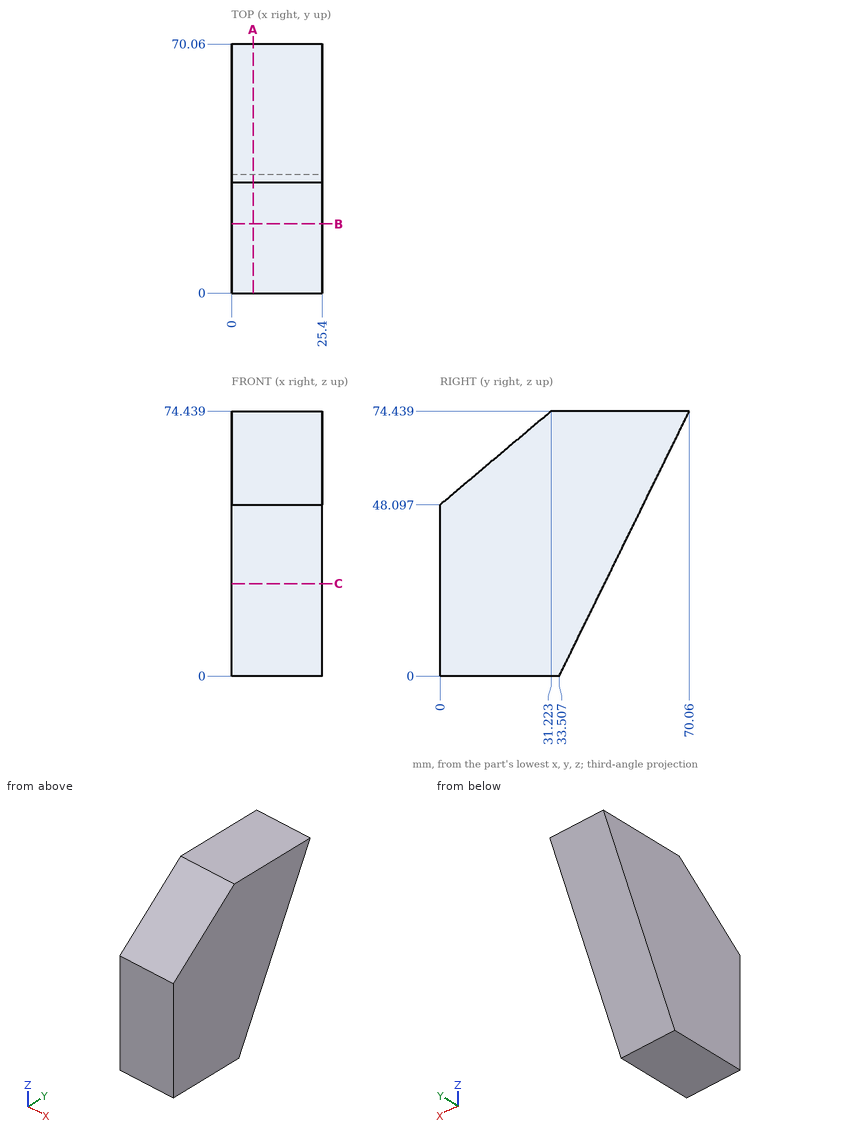
Could you check a few things on this drawing? It's one solid part, dimensions in mm from its lowest x, y, z. Give positions to 0.01 mm unless a question says otherwise; leave off trailing zeros. Order: outer loops, then holes, each group sorted by start corner. A loop starts at its lowest first (then second) coordinate and runs counter-clockwise, first axis right, second up.
1. Suppose I cut it at B-B (y = 19.5). Write out the boundary of the cut face in (x, z), plus the area to 3 significant figures.
Answers below:
outline: (0, 0) - (25.4, 0) - (25.4, 64.55) - (0, 64.55) - close
area: 1,640 mm2
2. I need wall thicknesses on L1, parallel to Y at x = 23.25, z = 37 (1 decimal); L2, parallel to Z at x = 2, y = 63 (1 decimal); L3, parallel to Y at x = 18.75, z = 4. Which ranges of each line are inside material? Lowest first, please.
Answers below:
L1: y = 0 to 51.7
L2: z = 60.1 to 74.4
L3: y = 0 to 35.47
3. Suppose I cut it at C-C (z = 26). Write out the boundary of the cut face in (x, y) (1 decimal).
Answers below:
outline: (0, 0) - (25.4, 0) - (25.4, 46.3) - (0, 46.3) - close
4. For pin 1 (6 mm diameter, centred on x = 8.5, y = 41.5, fed in from -Z) (1 decimal); pin 2 (1.5 mm diameter, centred on x = 21.5, y = 10.5, fed in from +Z); pin 3 (12 mm diameter, centred on x = 7, y = 41.5, fed in from -Z) (1 decimal), each with a flat end and sliding along its axis, tell me the tip position at first contact or that it passes through.
Answers below:
pin 1: stops at z = 10.2
pin 2: stops at z = 57.59
pin 3: stops at z = 4.1
5. Suppose I cut it at A-A (x = 6). Write out the boundary of the cut face in (y, z).
Answers below:
outline: (0, 0) - (33.51, 0) - (70.06, 74.44) - (31.22, 74.44) - (0, 48.1) - close
